Geometry: final body of the model. Coordinates: model frame, mm. A direction names the side the tool comes from. Round coordinates to 2 decimals unless told otherwise and drop trailing zeros. Loops run counter-clockwise (first coordinate to the right, second up) from the corner with the lowest first, then second, coordinate; pieces in that order, holes last. Notation, with made-up numbers: (-1, 42.25) - (51, 42.25) arc R22 ccw to (51, 49.25) - close; hole circle Ø11 at (-22.5, 32.25). An arc over 180 degrees is marked (long way). Return JSON: item names as keys, results as strings. Group by question number.
1. Section C-C on x = 0.8. Return loops of the section in (y, z).
2. First-contact query: pin 1 Ø0.5 at (y, z) = (1, -2.5) entering from +X (3 decimals); pin 2 Ø0.5 at (x, y) = (2.5, 2) entering from +Z (3 decimals); pin 3 Ø0.5 at (x, y) = (2.5, 7.5) entering from -Z (3 decimals). Flat tips, straight axial feed; report the tip coordinate or a pass-through.
3. Material intervals for probe 1 along Z at (x, y) = (0.15, 7.5) (3 decimals); probe 2 along X at (y, z) = (10.5, -7.75) (3 decimals); probe 3 along Y at (x, z) = (1, -8), sorted ascending.
4. Section D-D on y = 2.25. Count the separate pieces of the cut face and the enclosed holes in it, and give its area (3 significant figures).
5. Set-up query: faces 1 (the face through (1, 5.5, -4)), 2 (the face through (1, 3, -4)), 3 (the face through (3.81, 4, 0)). Return all of +Z, -Z, +X, -X, +Y, -Y with unobstructed straight access to the full face (end or side cutting, diameter ignored); none if empty.
6. Section B-B on z = -5. Return loops of the section in (x, y) (3 decimals).
7. Section A-A on y = 5. Return loops of the section in (x, z).
from build123d import *

# Parameters (mm, degrees)
EXTRUDE_1_DEPTH        = 12
PATTERN_LINEAR_1_COUNT = 2
PATTERN_LINEAR_1_PITCH = 2.54
EXTRUDE_2_DEPTH        = 2.5
PATTERN_LINEAR_2_COUNT = 4
PATTERN_LINEAR_2_PITCH = 2.54


with BuildPart() as part:
    # Sketch 1 → Extrude 1 (new body)
    with BuildSketch(Plane(origin=(0, 0, 0), x_dir=(1, 0, 0), z_dir=(0, 1, 0))):
        Polygon((-0.225, -0.325), (-0.325, -0.225), (-0.325, 0.225), (-0.225, 0.325), (0.225, 0.325), (0.325, 0.225), (0.325, -0.225), (0.225, -0.325), align=None)
    extrude(amount=EXTRUDE_1_DEPTH)


with BuildPart() as pattern_linear_1_1:
    # Pattern Linear 1: pattern copy
    add(part.part.moved(Location(Vector(1, 0, 0) * (1 * PATTERN_LINEAR_1_PITCH))))


with BuildPart() as part_1:
    add(part.part)

    add(pattern_linear_1_1.part)  # Extrude 2 merges Pattern Linear 1_1
    # Sketch 2 → Extrude 2 (add)
    with BuildSketch(Plane(origin=(0, 3, 0), x_dir=(-1, 0, 0), z_dir=(0, -1, 0))):
        Polygon((-3.31, 1.27), (-3.81, 0.77), (-3.81, -0.77), (-3.31, -1.27), (0.77, -1.27), (1.27, -0.77), (1.27, 0.77), (0.77, 1.27), align=None)
    extrude(amount=-EXTRUDE_2_DEPTH)


with BuildPart() as pattern_linear_2_1:
    # Pattern Linear 2: pattern copy
    add(part_1.part.moved(Location(Vector(0, 0, -1) * (1 * PATTERN_LINEAR_2_PITCH))))


with BuildPart() as pattern_linear_2_2:
    # Pattern Linear 2: pattern copy
    add(part_1.part.moved(Location(Vector(0, 0, -1) * (2 * PATTERN_LINEAR_2_PITCH))))


with BuildPart() as pattern_linear_2_3:
    # Pattern Linear 2: pattern copy
    add(part_1.part.moved(Location(Vector(0, 0, -1) * (3 * PATTERN_LINEAR_2_PITCH))))


with BuildPart() as part_2:
    add(part_1.part)

    # Combine 1: union Pattern Linear 2_1, Pattern Linear 2_2, Pattern Linear 2_3
    add(pattern_linear_2_1.part)
    add(pattern_linear_2_2.part)
    add(pattern_linear_2_3.part)


solid = part_2.part
Taken from the geometry:
{
 "1": {"outline": "(3, -8.89) - (5.5, -8.89) - (5.5, 1.27) - (3, 1.27) - close"},
 "2": {"pin 1": "x = 2.865", "pin 2": "z = 0.325", "pin 3": "z = -7.945"},
 "3": {"probe 1": "-7.945 to -7.295, -5.405 to -4.755, -2.865 to -2.215, -0.325 to 0.325", "probe 2": "-0.325 to 0.325, 2.215 to 2.865", "probe 3": "3 to 5.5"},
 "4": {"separate pieces": "8", "enclosed holes": "0", "area": "3.22 mm2"},
 "5": {"face 1": "+Y", "face 2": "-Y", "face 3": "+Z, -Z, +X, +Y, -Y"},
 "6": {"outline": "(-1.27, 3) - (-0.325, 3) - (-0.325, 0) - (0.325, 0) - (0.325, 3) - (2.215, 3) - (2.215, 0) - (2.865, 0) - (2.865, 3) - (3.81, 3) - (3.81, 5.5) - (2.865, 5.5) - (2.865, 12) - (2.215, 12) - (2.215, 5.5) - (0.325, 5.5) - (0.325, 12) - (-0.325, 12) - (-0.325, 5.5) - (-1.27, 5.5) - close"},
 "7": {"outline": "(-1.27, -8.39) - (-0.77, -8.89) - (3.31, -8.89) - (3.81, -8.39) - (3.81, -6.85) - (3.31, -6.35) - (3.81, -5.85) - (3.81, -4.31) - (3.31, -3.81) - (3.81, -3.31) - (3.81, -1.77) - (3.31, -1.27) - (3.81, -0.77) - (3.81, 0.77) - (3.31, 1.27) - (-0.77, 1.27) - (-1.27, 0.77) - (-1.27, -0.77) - (-0.77, -1.27) - (-1.27, -1.77) - (-1.27, -3.31) - (-0.77, -3.81) - (-1.27, -4.31) - (-1.27, -5.85) - (-0.77, -6.35) - (-1.27, -6.85) - close"}
}
